Can you work these out from the model? Positions are in its coordinate system, mm. Face numbers are marked on the shaded views. A direction names the side the tool comes from. Round coordinates to 2 decimals unless told otherwise and drop trailing zeros. Write each loop counter-clockwise with the first axis right and the second up, starting at its lowest first coordinate (ties: lowest second). Pieces come first, ordered by that corner, then holes.
Q1. If we section it at C-C (z = -23): Please give me the cut outline in (x, y) (3 decimals), plus the area to 3 significant figures.
Q2. For the marked faces 1, 2 and 3, which set-ups out of +Z, -Z, +X, -X, +Y, -Y let a thin tool reach every point of the face, with its end or its side?
Q3. If we section it at A-A (y = -47.5): Please give me the cut outline in (x, z), plus the area to 3 significant figures.
Q4. If we section it at D-D (y = -29): Please give me the cut outline in (x, z).
Q5. I'm going to push flat-ended pins straight in: pin 1 Ø3 at (x, z) = (-53, -6) entering from +Y; pin 2 Ø9.5 at (x, z) = (-42.5, -12.5) entering from -Y; pin 3 Ø15.5 at (x, z) = (-17.5, -12.5) entering from +Y. Where does each tip first touch, or does it pass through?
Q6. If we section it at B-B (z = -12.5): Give the number of separate pieces and of enclosed holes in the cut face, plus the area to 3 significant figures.
Q7. Please list where these lines run through material, in increasing order: line 1 along Z through (x, y) = (-7, -18.75); line 2 along X through (y, z) = (-24, -12.5); line 3 along Z through (x, y) = (-42, -5).
Q8. We'd pull the mould along X, two halves only. Please class the marked faces 4, 5 and 6: +X half, -X half, draft (parallel to the pull), parting line (faces both ways), or undercut.
Autodesk Inventor part; units mm, degrees
ref_plane "YZ Plane" through (0, 0, 0) normal (1, 0, 0) x (0, 1, 0)
ref_plane "XZ Plane" through (0, 0, 0) normal (0, 1, 0) x (-1, 0, 0)
ref_plane "XY Plane" through (0, 0, 0) normal (0, 0, 1) x (1, 0, 0)
sketch "Sketch1" plane through (0, 0, 0) normal (0, 1, 0) x (-1, 0, 0)
  line L0 (0, 0) -> (60, 0) construction
  line L1 (60, 0) -> (60, -25) construction
  line L2 (60, -25) -> (0, -25) construction
  line L3 (0, -25) -> (0, 0) construction
  line L4 (60.5, 0.5) -> (-0.5, 0.5)
  line L5 (-0.5, 0.5) -> (-0.5, -25.5)
  line L6 (-0.5, -25.5) -> (60.5, -25.5)
  line L7 (60.5, -25.5) -> (60.5, 0.5)
  circle A0 centre (53, -19) radius 1.8
  circle A1 centre (7, -19) radius 1.8
  circle A2 centre (7, -6) radius 1.8
  circle A3 centre (53, -6) radius 1.8
  line L8 (53, -19) -> (7, -19) construction
  line L9 (7, -19) -> (7, -6) construction
  point P0 (30, -19)
  point P1 (30, -25)
  point P2 (7, -12.5)
  point P3 (0, -12.5)
  dimension "d0" = 25
  dimension "d1" = 60
  dimension "d2" = 0.5
  dimension "d3" = 0.5
  dimension "d4" = 0.5
  dimension "d5" = 0.5
  dimension "d6" = 3.6
  dimension "d7" = 46
  dimension "d8" = 13
sketch "Sketch2" plane through (0, 0, 0) normal (0, 1, 0) x (-1, 0, 0)
  line L0 (-10, 5) -> (96.2, 5)
  line L1 (96.2, 5) -> (96.2, -30)
  line L2 (96.2, -30) -> (-10, -30)
  line L3 (-10, -30) -> (-10, 5)
  line L4 (60.5, -25.5) -> (60.5, 0.5) construction
  line L5 (-0.5, 0.5) -> (-0.5, -25.5) construction
  line L6 (-0.5, -25.5) -> (60.5, -25.5) construction
  point P0 (0, 0)
  point P1 (60.5, -12.5)
  point P2 (96.2, -12.5)
  point P3 (30, -25.5)
  point P4 (43.1, -30)
  point P5 (-10, -12.5)
  dimension "d9" = 106.2
  dimension "d10" = 35
  dimension "d51" = 10
extrude "Extrusion1" add sketch "Sketch2" along normal blind 10 and the other way blind 38.4
extrude "Extrusion2" cut sketch "Sketch1" along normal blind 10 and the other way blind 2
extrude "Extrusion3" cut sketch "Sketch1" along normal blind 10 and the other way blind 30.4 contours A0 | A1 | A2 | A3
sketch "Sketch3" plane through (10, 10, -30) normal (0, 0, -1) x (-1, 0, 0)
  line L0 (106.2, -48.4) -> (0, -48.4)
  line L1 (0, -48.4) -> (0, -78.4)
  line L2 (0, -78.4) -> (20, -78.4)
  line L3 (20, -78.4) -> (20, -51.575)
  line L4 (23.175, -48.4) -> (93.025, -48.4)
  line L5 (96.2, -51.575) -> (96.2, -78.4)
  line L6 (96.2, -78.4) -> (106.2, -78.4)
  line L7 (106.2, -78.4) -> (106.2, -48.4)
  arc A0 (23.175, -48.4) -> (20, -51.575) centre (23.175, -51.575) ccw
  arc A1 (96.2, -51.575) -> (93.025, -48.4) centre (93.025, -51.575) ccw
  point P0 (10, -10)
  point P1 (20, -48.4)
  point P2 (96.2, -48.4)
  point P3 (53.1, -48.4)
  point P4 (93.025, -48.4)
  dimension "d23" = 76.2
  dimension "d24" = 3.175
  dimension "d25" = 20
  dimension "d26" = 30
extrude "Extrusion4" add sketch "Sketch3" against normal up to surface (35 mm away)
sketch "Sketch4" plane through (0, -2, 0) normal (0, 1, 0) x (1, 0, 0)
  circle A0 centre (-42.5, 12.5) radius 3
  circle A1 centre (-17.5, 12.5) radius 3
  line L0 (-60.5, 25.5) -> (0.5, 25.5) construction
  line L1 (-60.5, -0.5) -> (-60.5, 25.5) construction
  line L2 (-42.5, 12.5) -> (-17.5, 12.5) construction
  point P0 (0, 0)
  point P1 (-30, 25.5)
  point P2 (-30, 12.5)
  point P3 (-60.5, 12.5)
  dimension "d29" = 6
  dimension "d30" = 25
extrude "Extrusion5" cut sketch "Sketch4" against normal up to surface (36.4 mm away)
sketch "Sketch5" plane through (0, -2, 0) normal (0, 1, 0) x (1, 0, 0)
  circle A0 centre (-42.5, 12.5) radius 3 construction
  circle A1 centre (-17.5, 12.5) radius 3 construction
  circle A2 centre (-17.5, 12.5) radius 6
  circle A3 centre (-42.5, 12.5) radius 6
  point P0 (0, 0)
  dimension "d34" = 12
extrude "Extrusion6" cut sketch "Sketch5" against normal blind 10
fillet "Fillet1" radius 2 2 edges at (-96.2, 10, -12.5) (10, 10, -12.5)
fillet "Fillet2" radius 2 2 edges at (-96.2, -68.4, -12.5) (10, -68.4, -12.5)
sketch "Sketch6" plane through (-83.025, -38.4, 5) normal (0, 0, 1) x (1, 0, 0)
  line L0 (69.85, 0) -> (0, 0) construction
  line L1 (35.525, 34.9) -> (70.525, 34.9)
  line L2 (69.85, 0) -> (0, 0)
  line L3 (-11.175, 48.4) -> (91.025, 48.4)
  line L4 (70.525, 34.9) -> (70.525, 48.4)
  line L5 (35.525, 34.9) -> (35.525, 48.4)
  line L6 (93.025, -28) -> (93.025, 46.4)
  point P0 (83.025, 38.4)
  point P1 (53.025, 34.9)
  point P2 (34.925, 0)
  point P3 (70.325, 0)
  point P4 (-0.475, 0)
  dimension "d39" = 34.9
  dimension "d40" = 35
  dimension "d50" = 40
extrude "Extrusion7" cut sketch "Sketch6" against normal up to surface (4.5 mm away)
sketch "Sketch7" plane through (-10, -68.4, -30) normal (0, 0, -1) x (-1, 0, 0)
  arc A0 (-2.9129, 78.4) -> (42.9129, 78.4) centre (20, 88.4) ccw
  line L0 (-18, 78.4) -> (84.2, 78.4)
  point P0 (-10, 68.4)
  point P1 (33.1, 78.4)
  point P2 (-20, 76.4)
  dimension "d44" = 25
  dimension "d45" = 10
  dimension "d49" = 40
extrude "Extrusion8" cut sketch "Sketch7" against normal blind 10
properties part number "BK12_Spacer"
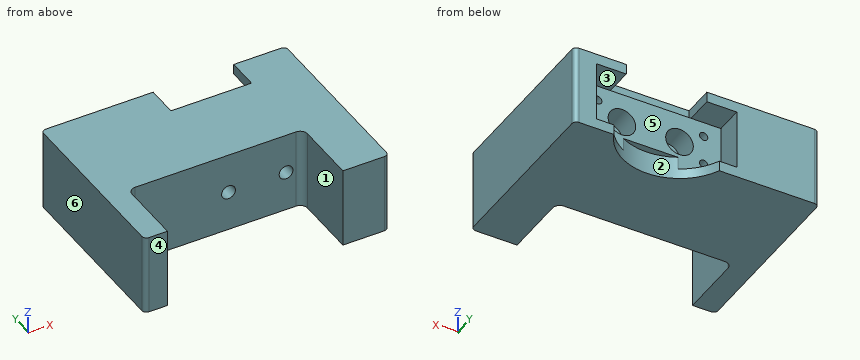
A:
1. outline: (-96.2, -66.4) arc R2 ccw to (-94.2, -68.4) - (-86.2, -68.4) - (-86.2, -41.575) arc R3.175 cw to (-83.025, -38.4) - (-13.175, -38.4) arc R3.175 cw to (-10, -41.575) - (-10, -68.4) - (8, -68.4) arc R2 ccw to (10, -66.4) - (10, 8) arc R2 ccw to (8, 10) - (0.5, 10) - (0.5, -2) - (-18.126, -2) arc R25 cw to (-41.874, -2) - (-60.5, -2) - (-60.5, 10) - (-94.2, 10) arc R2 ccw to (-96.2, 8) - close
1. area: 5,260 mm2
2. face 1: +Z, -Z, -Y
2. face 2: -Z, +Y
2. face 3: +Y
3. outline: (-96.2, -30) - (-86.2, -30) - (-86.2, 5) - (-96.2, 5) - close; (-10, -30) - (10, -30) - (10, 5) - (-10, 5) - close
3. area: 1,050 mm2
4. outline: (-96.2, -30) - (10, -30) - (10, 5) - (-96.2, 5) - close; hole circle Ø3.6 at (-53, -19); hole circle Ø3.6 at (-53, -6); hole circle Ø6 at (-42.5, -12.5); hole circle Ø6 at (-17.5, -12.5); hole circle Ø3.6 at (-7, -19); hole circle Ø3.6 at (-7, -6)
5. pin 1: stops at y = -30.4
5. pin 2: stops at y = -38.4
5. pin 3: stops at y = -2
6. separate pieces: 3
6. enclosed holes: 0
6. area: 4,750 mm2
7. line 1: z = -30 to -20.8, -17.2 to -7.8, -4.2 to 5
7. line 2: x = -96.2 to -45.5, -39.5 to -20.5, -14.5 to 10
7. line 3: z = -30 to -18.48, -6.52 to 5
8. face 4: draft
8. face 5: undercut
8. face 6: -X half
